Geometry check sheet. Reference: drawing and pictorial views, mm from the part's lowest x, y, z. Round coordinates to 2 decimals unless told otherwise and drop trailing zeros. Order: outer loops, then holes, each group sorted by start corner. A loop starts at its lowest first (then second) coordinate and runs counter-clockwise, first axis right, second up.
Q1. Cross-section at A-A on z = 8.5. Record the cut outline in (x, y).
Q2. Cross-section at B-B on z = 14.25. Record the cut outline in (x, y).
Q3. Scan lines: probe 1 along Y at (x, z) = (20, 7.75); probe 2 along Y at (x, z) = (23, 2); probe 3 along X at (y, z) = (17.5, 1.75) (1 decimal). Record each from-to range of solid material in increasing order.
Q4. Mould release check, pull along X, two halves, no side actions. Record for the marked faces 1, 2 and 3: +X half, -X half, draft (parallel to the pull), parting line (faces both ways), or undercut.
Q5. Depth check by flat-ended pin: P1, Ø5, axis at y = 14.5, z = 3, coming from the +X side (1 decimal); P2, Ø1.5, axis at y = 19.5, z = 12, coming from the -X side (1 decimal); P3, Ø4, axis at y = 26, z = 3, coming from the +X side. Enter the tip coordinate at first touch or a pass-through.
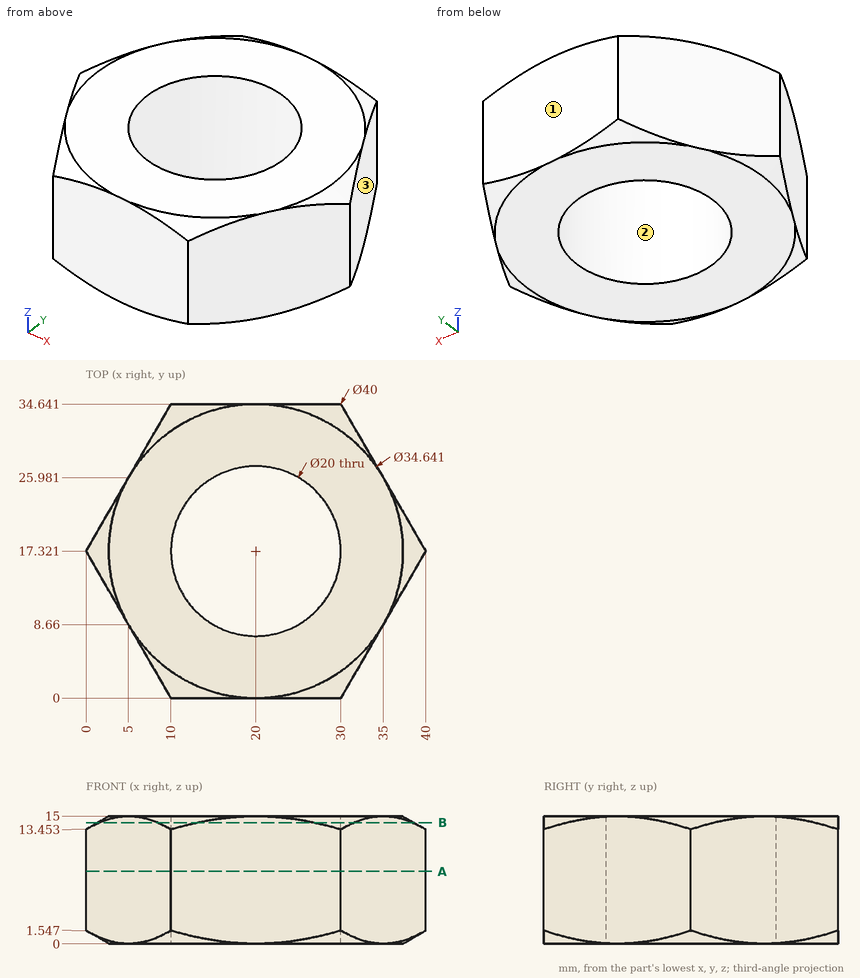
Results found:
1. outline: (0, 17.32) - (10, 0) - (30, 0) - (40, 17.32) - (30, 34.64) - (10, 34.64) - close; hole circle Ø20 at (20, 17.32)
2. outline: (1.58, 14.58) - (8.42, 2.74) arc R18.62 ccw to (13.17, 0) - (26.83, 0) arc R18.62 ccw to (31.58, 2.74) - (38.42, 14.58) arc R18.62 ccw to (38.42, 20.06) - (31.58, 31.9) arc R18.62 ccw to (26.83, 34.64) - (13.17, 34.64) arc R18.62 ccw to (8.42, 31.9) - (1.58, 20.06) arc R18.62 ccw to start; hole circle Ø20 at (20, 17.32)
3. probe 1: y = 0 to 7.32, 27.32 to 34.64
3. probe 2: y = 0 to 7.78, 26.86 to 34.64
3. probe 3: x = 0.1 to 10, 30 to 39.9
4. face 1: draft
4. face 2: undercut
4. face 3: +X half
5. P1: stops at x = 39.8
5. P2: stops at x = 0.8
5. P3: stops at x = 36.14
